Read the model definition and answer for the solid it produces. Units are mm, in the model's axes. Face numbers are marked on the shaded views. A direction names the side the tool comes from. Coordinates: 2 decimals unless noted, no trailing zeros. Loops run counter-clockwise (first coordinate to the right, second up) from the corner with the lowest first, then second, coordinate; pieces in that order, holes last. Notation, with made-up numbers: (12.5, -1.75) - (69.5, -1.75) arc R10 ccw to (69.5, 14.25) - close; hole circle Ø8 at (25.5, 12). An arc over 180 degrees is marked (long way). One line per question, with ' | ' between items. Start each with the question number.
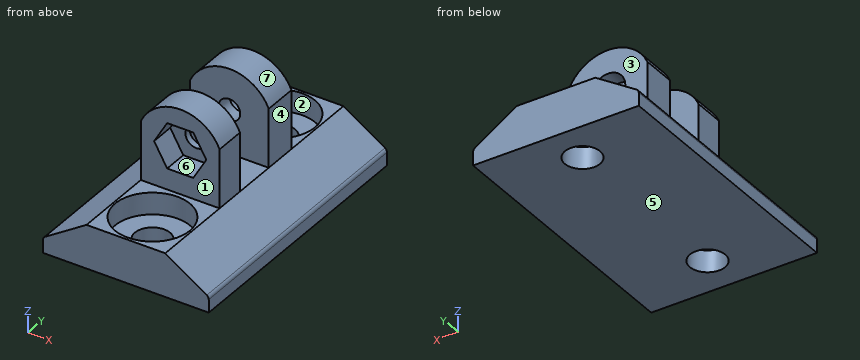
```python
from build123d import *

# Parameters (mm, degrees)
PAD_DEPTH         = 62
SKETCH003_R       = 4.05
POCKET_DEPTH      = 0.001
POCKET_DEPTH_BACK = -10.001
SKETCH_R          = 8.625
POCKET001_DEPTH   = 5
PAD001_DEPTH      = 25
BOX_W             = 20
BOX_H             = 20
BOX_DEPTH         = 10
SKETCH005_R       = 2.5
POCKET002_DEPTH   = 62.001
CYLINDER_R        = 4
CYLINDER_DEPTH    = 4
POCKET003_DEPTH   = 6


with BuildPart() as part:
    # Sketch002 (on Sketch) → Pad (new body)
    with BuildSketch(Plane.XZ):
        with BuildLine():
            Line((-38.1, 3), (-38.1, 0))
            Line((-38.1, 0), (0, 0))
            Line((0, 3), (0, 0))
            ThreePointArc((0, 3), (-0.121836, 3.47836), (-0.457656, 3.840157))
            Line((-10, 10), (-0.457656, 3.840157))
            Line((-28.1, 10), (-10, 10))
            Line((-28.1, 10), (-37.642344, 3.840157))
            ThreePointArc((-37.642344, 3.840157), (-37.978164, 3.47836), (-38.1, 3))
        make_face()
    extrude(amount=PAD_DEPTH)

    # Sketch003 → Pocket (cut, two sides)
    with BuildSketch(Plane.XY) as pocket_sk:
        with Locations((-19.05, -9.25)):
            Circle(SKETCH003_R)
        with Locations((-19.05, -52.75)):
            Circle(SKETCH003_R)
    extrude(amount=-POCKET_DEPTH, mode=Mode.SUBTRACT)
    extrude(pocket_sk.sketch, amount=-POCKET_DEPTH_BACK, mode=Mode.SUBTRACT)

    # Sketch → Pocket001 (cut)
    with BuildSketch(Plane.XY.offset(5)):
        with Locations((-19.05, -9.25)):
            Circle(SKETCH_R)
        with Locations((-19.05, -52.75)):
            Circle(SKETCH_R)
    extrude(amount=POCKET001_DEPTH, mode=Mode.SUBTRACT)

    # Sketch004 → Pad001 (join)
    with BuildSketch(Plane.XZ.offset(18.1)):
        with BuildLine():
            Line((-28.1, 10), (-10, 10))
            Line((-10, 23.5), (-10, 10))
            ThreePointArc((-10, 23.5), (-19.05, 29.402761), (-28.1, 23.5))
            Line((-28.1, 10), (-28.1, 23.5))
        make_face()
    extrude(amount=PAD001_DEPTH)

    # Box → Box (cut)
    with BuildSketch(Plane(origin=(-29, -26, 10), x_dir=(1, 0, 0), z_dir=(0, -1, 0))):
        with Locations((10, 10)):
            Rectangle(BOX_W, BOX_H)
    extrude(amount=BOX_DEPTH, mode=Mode.SUBTRACT)

    # Sketch005 → Pocket002 (cut, through all)
    with BuildSketch(Plane.XZ):
        with Locations((-19.05, 20)):
            Circle(SKETCH005_R)
    extrude(amount=POCKET002_DEPTH, mode=Mode.SUBTRACT)

    # Cylinder → Cylinder (cut)
    with BuildSketch(Plane(origin=(-19.05, -22.1, 20), x_dir=(0, 0, -1), z_dir=(0, 1, 0))):
        Circle(CYLINDER_R)
    extrude(amount=CYLINDER_DEPTH, mode=Mode.SUBTRACT)

    # Sketch006 → Pocket003 (cut)
    with BuildSketch(Plane.XZ.offset(37.5)):
        Polygon((-16.05, 25.196152), (-22.05, 25.196152), (-25.05, 20), (-22.05, 14.803848), (-16.05, 14.803848), (-13.05, 20), align=None)
    extrude(amount=POCKET003_DEPTH, mode=Mode.SUBTRACT)


solid = part.part
```
1) Find the intervals of material crossed by line 1 along Y through (x, z) = (-19.05, 6.55) (3 decimals); line 2 along Y through (x, z) = (-19.05, 3.4); line 3 along Y through (x, z) = (-23, 12), in increasing order. Write a range as from..to.
2) The mould has two halves that part along X. Classify the marked faces 5, 6 and 7: released by +X, released by -X, zero draft, split by the parting line, or undercut.
3) The part is cut by section A-A on y = -52.75. Write down the section's boundary in (x, z) (3 decimals).
4) Given pin 1 Ø6.5 at (x, z) = (-19.05, 20) entering from -Y; pin 2 Ø5.5 at (x, y) = (-18, -54.5) entering from +Z; pin 3 Ø5.5 at (x, z) = (-20, 24.5) entering from +Y, each flat-ended and moving along its own axis, determine where each tip first touches the part or whether it passes through.
5) The part is cut by section C-C on y = -25. Write down the section's boundary in (x, z).
6) The part is cut by section D-D on x = -14. Write down the section's boundary in (y, z), and give its area (3 significant figures).
7) The part is cut by section B-B on z = 11.25. Write down the section's boundary in (x, y).
8) Which of the six approach directions +Z, -Z, +X, -X, +Y, -Y give full straight-line access (tool end or side, diameter ignored) to the marked faces 1, 2, 3 and 4?
Answer below:
1) line 1: -62..-61.375, -44.125..-17.875, -0.625..0 | line 2: -62..-56.8, -48.7..-13.3, -5.2..0 | line 3: -43.1..-36, -26..-18.1
2) face 5: zero draft | face 6: undercut | face 7: split by the parting line
3) outline: (-38.1, 0) - (-23.1, 0) - (-23.1, 5) - (-27.675, 5) - (-27.675, 10) - (-28.1, 10) - (-37.642, 3.84) arc R1 ccw to (-38.1, 3) - close; (-15, 0) - (0, 0) - (0, 3) arc R1 ccw to (-0.458, 3.84) - (-10, 10) - (-10.425, 10) - (-10.425, 5) - (-15, 5) - close
4) pin 1: y = -37.5 | pin 2: z = 5 | pin 3: y = -18.1
5) outline: (-38.1, 0) - (0, 0) - (0, 3) arc R1 ccw to (-0.46, 3.84) - (-10, 10) - (-10, 23.5) arc R9.89 ccw to (-28.1, 23.5) - (-28.1, 10) - (-37.64, 3.84) arc R1 ccw to (-38.1, 3) - close; hole circle Ø5 at (-19.05, 20)
6) outline: (-62, 0) - (0, 0) - (0, 10) - (-2.26, 10) - (-2.26, 5) - (-16.24, 5) - (-16.24, 10) - (-18.1, 10) - (-18.1, 28.02) - (-26, 28.02) - (-26, 10) - (-36, 10) - (-36, 28.02) - (-43.1, 28.02) - (-43.1, 21.65) - (-37.5, 21.65) - (-37.5, 18.35) - (-43.1, 18.35) - (-43.1, 10) - (-45.76, 10) - (-45.76, 5) - (-59.74, 5) - (-59.74, 10) - (-62, 10) - close | area: 732 mm2
7) outline: (-28.1, -43.1) - (-10, -43.1) - (-10, -36) - (-28.1, -36) - close; (-28.1, -26) - (-10, -26) - (-10, -18.1) - (-28.1, -18.1) - close
8) face 1: +Z, +X, -X, -Y | face 2: +Z | face 3: +Z, +X, -X, +Y | face 4: +Z, +X, +Y, -Y
